from build123d import *

# Parameters (mm, degrees)
SKETCH1_W           = 25.4
SKETCH1_H           = 76.2
BOSS_EXTRUDE1_DEPTH = 4.7625
SKETCH2_R           = 2.38125
CUT_EXTRUDE1_DEPTH  = 5.7625


with BuildPart() as part:
    # Sketch1 → Boss-Extrude1 (new body)
    with BuildSketch(Plane(origin=(0, 0, 0), x_dir=(1, 0, 0), z_dir=(0, 1, 0))):
        Rectangle(SKETCH1_W, SKETCH1_H)
    extrude(amount=BOSS_EXTRUDE1_DEPTH)

    # Sketch2 → Cut-Extrude1 (cut, through all)
    with BuildSketch(Plane(origin=(0, 4.7625, 0), x_dir=(1, 0, 0), z_dir=(0, 1, 0))):
        with Locations((0, 25.4)):
            Circle(SKETCH2_R)
        Circle(SKETCH2_R)
        with Locations((0, -25.4)):
            Circle(SKETCH2_R)
    extrude(amount=-CUT_EXTRUDE1_DEPTH, mode=Mode.SUBTRACT)


solid = part.part
Model file for the job. Use its own axes, mm. Give positions to 0.01 mm unless a question says otherwise; leave off trailing zeros. Write each loop counter-clockwise with the first axis right and the second up, starting at its lowest first coordinate (ties: lowest second). Pieces come first, ordered by that corner, then holes. Notation, with made-up numbers: (-4, 58.5) -> (4, 58.5) arc R15 ccw to (4, 66.5) -> close; hole circle Ø11 at (69, 50). An arc over 180 degrees is marked (long way). Write item = value, one per line.
(1) Slice it at A-A, the plane y = 2. Give the cut face in (x, z), then the cut area to 3 significant figures.
Determined:
outline = (-12.7, -38.1) -> (12.7, -38.1) -> (12.7, 38.1) -> (-12.7, 38.1) -> close; hole circle Ø4.76 at (0, -25.4); hole circle Ø4.76 at (0, 0); hole circle Ø4.76 at (0, 25.4)
area = 1,880 mm2
(2) Slice it at C-C, the plane x = -0.75. Give the cut face in (y, z).
Determined:
outline = (0, -38.1) -> (4.76, -38.1) -> (4.76, -27.66) -> (0, -27.66) -> close; (0, -23.14) -> (4.76, -23.14) -> (4.76, -2.26) -> (0, -2.26) -> close; (0, 2.26) -> (4.76, 2.26) -> (4.76, 23.14) -> (0, 23.14) -> close; (0, 27.66) -> (4.76, 27.66) -> (4.76, 38.1) -> (0, 38.1) -> close
(3) Slice it at B-B, the plane z = 25.4. Give the cut face in (x, y), then the cut area to 3 significant figures.
Determined:
outline = (-12.7, 0) -> (-2.38, 0) -> (-2.38, 4.76) -> (-12.7, 4.76) -> close; (2.38, 0) -> (12.7, 0) -> (12.7, 4.76) -> (2.38, 4.76) -> close
area = 98.3 mm2
(4) Mould opens along Z. For faces 1 (the face through (-1.755, 2.415, -27.009)), 2 (the face through (0, 2, -38.1)), 3 (the face through (-12.7, 2, 1)) say: released by +Z, released by -Z, zero draft, split by the parting line, or undercut.
Determined:
face_1 = undercut
face_2 = released by -Z
face_3 = zero draft
(5) Probe line 1 along Z through (x, y) = (0, 2.85); line 2 along X through (y, z) = (2, 0); line 3 along Z through (x, y) = (1.5, 2.8). List the from-to ranges inside material, lowest first.
Determined:
line_1 = -38.1 to -27.78, -23.02 to -2.38, 2.38 to 23.02, 27.78 to 38.1
line_2 = -12.7 to -2.38, 2.38 to 12.7
line_3 = -38.1 to -27.25, -23.55 to -1.85, 1.85 to 23.55, 27.25 to 38.1
